Source: CAD feature listing. Evaluate the final solid. Frame: model axes, mm. Face numbers are marked on the shaded views. Coordinates: 2 decimals unless noted, no trailing zeros. Order: outer loops, then holes, each group sorted by start corner. A loop starts at its lowest first (then second) coordinate and runs counter-clockwise, first axis right, second up.
Item 1: Section C-C on x = -33.5. Return the cut outline in (y, z), then the cut area to 3 significant figures.
Item 2: Section B-B on z = 6. Return the cut outline in (x, y).
Item 3: Ray query, line 1 (X direction, y = 0, z = -8.3); line 2 (Z direction, x = -21, y = 0); line 3 (Y direction, x = -13.5, z = 6). Return the intervals inside material, ascending.
Item 4: Section A-A on y = 0. Return the cut outline in (x, z), then the cut area to 3 significant figures.
Item 5: Section D-D on x = -10. Return the cut outline in (y, z), then the cut area to 3 significant figures.
Item 6: Mould query, pull axis Y, two halves, no side actions, for the marked faces 1 and 2. Classes: released by +Y, released by -Y, zero draft, split by the parting line, or undercut.
Item 7: Contact query for flat-ended pins moving along their axis: P1, Ø3, axis at x = -7.5, y = 0, coming from the -Z side; P2, Ø3, axis at x = -25.5, y = 4, coming from the -Z side; P3, Ø2, axis at x = -7.5, y = 0, coming from the +Z side; P4, Ø3, axis at x = -33.5, y = 6.5, coming from the +Z side. Output: stop coordinate, or through.
Autodesk Inventor part; units mm, degrees
ref_plane "MidSidePlane" through (0, 0, 10) normal (0, 0, 1) x (1, 0, 0)
ref_plane "YZ Plane" through (0, 0, 0) normal (1, 0, 0) x (0, 1, 0)
ref_plane "XZ Plane" through (0, 0, 0) normal (0, 1, 0) x (-1, 0, 0)
sketch "ShaftProfile" plane through (0, 0, 0) normal (0, 0, 1) x (1, 0, 0)
  line L0 (-45.6, 0) -> (7.6, 0) construction
  line L1 (-38, 9) -> (-3, 9)
  line L2 (-3, 9) -> (-3, 0)
  line L3 (-38, 0) -> (-38, 9)
  line L4 (-38, 0) -> (-3, 0)
  point P0 (0, 0)
  dimension "d1" = 35
  dimension "d2" = 9
  dimension "d4" = 38
revolve "ShaftFeature" add sketch "ShaftProfile" angle 360 about axis through (-38, 0, 0) along (1, 0, 0)
sketch "Sketch2" plane through (-38, 0, 0) normal (-1, 0, 0) x (0, 0, 1)
  circle A0 centre (0, 0) radius 9
hole "ShaftHoleFeature" at (-38, 0, 0) direction (1, 0, 0) diameter 16 end through all
ref_plane "MidSidePlane" through (0, 0, 10) normal (0, 0, 1) x (1, 0, 0)
sketch "CapHoles" plane through (0, 0, 10) normal (0, 0, 1) x (1, 0, 0)
  line L0 (-3, -9) -> (-3, 9) construction
  line L1 (-38, -9) -> (-38, 9) construction
  line L2 (-48, 0) -> (22, 0) construction
  circle A0 centre (-33.5, 0) radius 1.25
  circle A1 centre (-7.5, 0) radius 1.25
  dimension "d24" = 2.5
  dimension "d25" = 4.5
  dimension "d26" = 4.5
extrude "CapHolesFeature" cut sketch "CapHoles" against normal through all
equation "\"d26\" = d25"
properties part number "BackPair1PistonShaft"
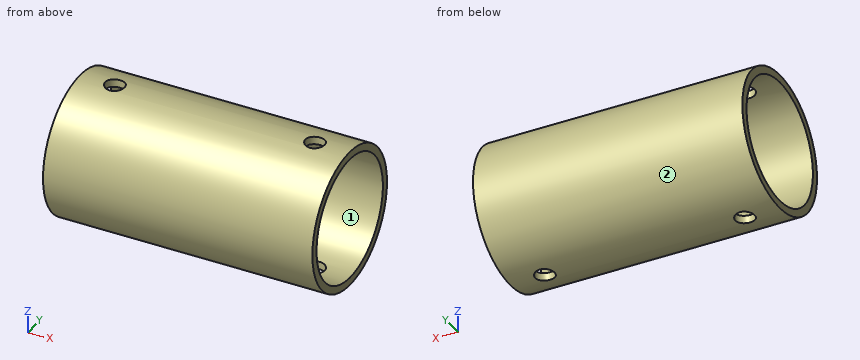
Answer list:
1. outline: (-1.25, -8.91) - (-1.25, -7.9) arc R8 cw to (-1.25, 7.9) - (-1.25, 8.91) arc R9 ccw to start; (1.25, -8.91) arc R9 ccw to (1.25, 8.91) - (1.25, 7.9) arc R8 cw to (1.25, -7.9) - close
1. area: 48.4 mm2
2. outline: (-38, -6.71) - (-3, -6.71) - (-3, -5.29) - (-38, -5.29) - close; (-38, 5.29) - (-3, 5.29) - (-3, 6.71) - (-38, 6.71) - close
3. line 1: x = -38 to -34.75, -32.25 to -8.75, -6.25 to -3
3. line 2: z = -9 to -8, 8 to 9
3. line 3: y = -6.71 to -5.29, 5.29 to 6.71
4. outline: (-38, -9) - (-34.75, -9) - (-34.75, -8) - (-38, -8) - close; (-38, 8) - (-34.75, 8) - (-34.75, 9) - (-38, 9) - close; (-32.25, -9) - (-8.75, -9) - (-8.75, -8) - (-32.25, -8) - close; (-32.25, 8) - (-8.75, 8) - (-8.75, 9) - (-32.25, 9) - close; (-6.25, -9) - (-3, -9) - (-3, -8) - (-6.25, -8) - close; (-6.25, 8) - (-3, 8) - (-3, 9) - (-6.25, 9) - close
4. area: 60.0 mm2
5. outline: circle Ø18 at (0, 0); hole circle Ø16 at (0, 0)
5. area: 53.4 mm2
6. face 1: undercut
6. face 2: split by the parting line
7. P1: stops at z = -9
7. P2: stops at z = -8.65
7. P3: passes through
7. P4: stops at z = 7.48
